Autodesk Inventor part; units mm, degrees
ref_plane "YZ Plane" through (0, 0, 0) normal (1, 0, 0) x (0, 1, 0)
ref_plane "XZ Plane" through (0, 0, 0) normal (0, 1, 0) x (-1, 0, 0)
ref_plane "XY Plane" through (0, 0, 0) normal (0, 0, 1) x (1, 0, 0)
sketch "Sketch1" plane through (0, 0, 0) normal (0, 0, 1) x (1, 0, 0)
  line L0 (0, 0) -> (12.7, 0)
  line L1 (12.7, 0) -> (12.7, 12.7)
  line L2 (12.7, 12.7) -> (0, 12.7)
  line L3 (0, 12.7) -> (0, 0)
  dimension "d0" = 12.7
  dimension "d1" = 12.7
extrude "Extrusion1" add sketch "Sketch1" along normal blind 5.08
sketch "Sketch3" plane through (0, 0, 5.08) normal (0, 0, 1) x (1, 0, 0)
  line L0 (3.81, 8.89) -> (8.89, 8.89)
  line L1 (8.89, 8.89) -> (8.89, 3.81)
  line L2 (8.89, 3.81) -> (3.81, 3.81)
  line L3 (3.81, 3.81) -> (3.81, 8.89)
  line L4 (0, 12.7) -> (0, 0)
  line L5 (12.7, 0) -> (12.7, 12.7)
  line L6 (12.7, 12.7) -> (0, 12.7)
  line L7 (0, 0) -> (12.7, 0)
  point P0 (12.7, 6.35)
  dimension "d10" = 3.81
  dimension "d11" = 3.81
  dimension "d12" = 3.81
  dimension "d13" = 3.81
extrude "Extrusion3" add sketch "Sketch3" along normal blind 5.08 contours L0 L1 L2 L3
properties part number "Handle"
Geometry check sheet. Reference: the model listing, model coordinates, mm. A direction names the side the tool comes from. Coordinates: 2 decimals unless noted, no trailing zeros. Write each loop counter-clockwise with the first axis right and the second up, starting at its lowest first coordinate (ties: lowest second). Pieces come first, ordered by that corner, then holes. Notation, with made-up numbers: M 87,71.25 L 131,71.25 A19 cw 131,93.25 Z; hole C 32,-36.5 d6. An arc over 180 degrees is marked long. One line per item, written item: value. Start each with the question number.
(1) Depth check by flat-ended pin: pin 1 (1 mm diameter, centred on x = 7.5, z = 6, fed in from +Y); pin 2 (3 mm diameter, centred on y = 4, z = 4.5, fed in from -X); pin 3 (2 mm diameter, centred on x = 10.5, z = 6.5, fed in from +Y); pin 4 (5.5 mm diameter, centred on x = 6.5, z = 8, fed in from -Y). Enter the tip coordinate at first touch or a pass-through.
(2) Tool access check on faces 1 (the face through (6, 8.89, 8)), 2 (the face through (3.81, 6, 8)), 3 (the face through (8.89, 6, 8)), 4 (the face through (6, 3.81, 8)). Record the directions out of +Z, -Z, +X, -X, +Y, -Y that give a thin tool (end or side, any length) a straight path to the whole face; none if there is none.
(3) Scan lines: line 1 along Y through (x, z) = (7.5, 8); line 2 along Z through (x, y) = (5.5, 0.75). Record each from-to range of solid material in increasing order. Write a range as [from, to].
(4) Sectioned sample at C-C, the plane z = 7.75. Enter the section's corners in (x, y), and give its area (3 significant figures).
(5) Sectioned sample at D-D, the plane x = 10.5. Enter the section's corners in (y, z).
(6) Sectioned sample at A-A, the plane x = 5. Enter the section's corners in (y, z).
Filled sheet:
1. pin 1: y = 8.89
1. pin 2: x = 0
1. pin 3: through
1. pin 4: y = 3.81
2. face 1: +Z, +X, -X, +Y
2. face 2: +Z, -X, +Y, -Y
2. face 3: +Z, +X, +Y, -Y
2. face 4: +Z, +X, -X, -Y
3. line 1: [3.81, 8.89]
3. line 2: [0, 5.08]
4. outline: M 3.81,3.81 L 8.89,3.81 L 8.89,8.89 L 3.81,8.89 Z
4. area: 25.8 mm²
5. outline: M 0,0 L 12.7,0 L 12.7,5.08 L 0,5.08 Z
6. outline: M 0,0 L 12.7,0 L 12.7,5.08 L 8.89,5.08 L 8.89,10.16 L 3.81,10.16 L 3.81,5.08 L 0,5.08 Z
